from build123d import *

# Parameters (mm, degrees)
SKETCH1_W           = 18.495
SKETCH1_H           = 20.8
SKETCH1_W_2         = 10
SKETCH1_W_3         = 37.395
BOSS_EXTRUDE1_DEPTH = 10
SKETCH2_W           = 10
SKETCH2_H           = 20.8
BOSS_EXTRUDE2_DEPTH = 28.2
SKETCH6_W           = 106.79
SKETCH6_H           = 10
BOSS_EXTRUDE4_DEPTH = 10
SKETCH9_R           = 2.35
CUT_EXTRUDE1_DEPTH  = 10


with BuildPart() as part:
    # Sketch1 → Boss-Extrude1 (new body)
    with BuildSketch(Plane.XY):
        with Locations((-39.1475, 0)):
            Rectangle(SKETCH1_W, SKETCH1_H)
        with Locations((-53.395, 0)):
            Rectangle(SKETCH1_W_2, SKETCH1_H)
        with Locations((29.6975, 0)):
            Rectangle(SKETCH1_W_3, SKETCH1_H)
    extrude(amount=BOSS_EXTRUDE1_DEPTH)

    # Sketch2 → Boss-Extrude2 (add)
    with BuildSketch(Plane.XY.offset(10)):
        with Locations((43.395, 0)):
            Rectangle(SKETCH2_W, SKETCH2_H)
        with Locations((-53.395, 0)):
            Rectangle(SKETCH2_W, SKETCH2_H)
    extrude(amount=BOSS_EXTRUDE2_DEPTH)

    # Sketch6 → Boss-Extrude4 (add)
    with BuildSketch(Plane(origin=(0, 10.4, 0), x_dir=(1, 0, 0), z_dir=(0, 1, 0))):
        with Locations((-5, -5)):
            Rectangle(SKETCH6_W, SKETCH6_H)
    extrude(amount=BOSS_EXTRUDE4_DEPTH)

    # Sketch9 → Cut-Extrude1 (cut)
    with BuildSketch(Plane.XY.offset(10)):
        with Locations((14.89, -4.9)):
            Circle(SKETCH9_R)
        with Locations(Location((14.89, 4.9, 0), (0, 0, 180))):
            Circle(SKETCH9_R)
        with Locations(Location((-33.79, -4.9, 0), (0, 0, 180))):
            Circle(SKETCH9_R)
        with Locations((-33.79, 4.9)):
            Circle(SKETCH9_R)
    extrude(amount=-CUT_EXTRUDE1_DEPTH, mode=Mode.SUBTRACT)


solid = part.part
Verification items for the finished model (mm, model axes). A direction names the side the tool comes from. Coordinates: 2 decimals unless noted, no trailing zeros. Order: outer loops, then holes, each group sorted by start corner. A loop starts at its lowest first (then second) coordinate and runs counter-clockwise, first axis right, second up. Notation, with made-up numbers: M -25,82.25 L 4,82.25 A14 ccw 4,98.25 Z; hole C 36,1 d7. An arc over 180 degrees is marked long. One line per item, written item: value. Start each with the question number.
Item 1: Scan lines: probe 1 along Y at (x, z) = (14.89, 6.25); probe 2 along Y at (x, z) = (14, 2); probe 3 along X at (y, z) = (-4, 6) (3 decimals). Record each from-to range of solid material in increasing order.
Item 2: Gauge pin test, flat ends, axial feed: pin 1 (3 mm diameter, centred on x = 43.5, z = 23.5, fed in from +Y); pin 2 (8 mm diameter, centred on x = -24.5, z = 16.5, fed in from -Y); pin 3 (15.5 mm diameter, centred on x = -3.5, y = 11, fed in from +Z); pin 4 (8 mm diameter, centred on x = -3.5, z = 7.5, fed in from -Y). Record the tip position at first contact, or that the pin passes through.
Item 3: Sectioned sample at C-C (x = 16). Enter the section's corners in (y, z), then the cut area to 3 significant figures.
Item 4: Access from +Z, -Z, +X, -X, +Y, -Y to the whole of each face (thin tool, end or side, straight path). Record for faces 4 (the flat face through (-53, 10.4, 24)), 5 (the flat face through (11, 0, 5)), 6 (the flat face through (-48.395, 0, 24)), 7 (the cylindrical face through (-31.62, 4, 5.07)).
Item 5: Mould release check, pull along X, two halves, no side actions. Record for faces 1 (the flat face through (-10, 10.4, 5)), 2 (the flat face through (-58.395, 1, 19)), 3 (the flat face through (-51, -10.4, 15)): released by +X, released by -X, zero draft, split by the parting line, or undercut.
Item 6: Sectioned sample at D-D (y = -4.9). Enter the section's corners in (x, z) (3 decimals), then the cut area to 3 significant figures.
Item 7: Sectioned sample at B-B (z = 3). Enter the section's corners in (x, y) (3 decimals).
Item 8: Sectioned sample at A-A (y = 9). Enter the section's corners in (x, z) (3 decimals), then the cut area to 3 significant figures.
Conclusion:
1. probe 1: y = -10.4 to -7.25, -2.55 to 2.55, 7.25 to 20.4
1. probe 2: y = -10.4 to -7.07, -2.73 to 2.73, 7.07 to 20.4
1. probe 3: x = -58.395 to -35.961, -31.619 to -29.9, 11 to 12.719, 17.061 to 48.395
2. pin 1: stops at y = 10.4
2. pin 2: passes through
2. pin 3: stops at z = 10
2. pin 4: stops at y = 10.4
3. outline: M -10.4,0 L -6.97,0 L -6.97,10 L -10.4,10 Z; M -2.83,0 L 2.83,0 L 2.83,10 L -2.83,10 Z; M 6.97,0 L 20.4,0 L 20.4,10 L 6.97,10 Z
3. area: 225 mm^2
4. face 4: +Z, +X, -X, +Y
4. face 5: +Z, -Z, -Y
4. face 6: +Z, +Y, -Y
4. face 7: +Z, -Z
5. face 1: undercut
5. face 2: released by -X
5. face 3: zero draft
6. outline: M -58.395,0 L -36.14,0 L -36.14,10 L -48.395,10 L -48.395,38.2 L -58.395,38.2 Z; M -31.44,0 L -29.9,0 L -29.9,10 L -31.44,10 Z; M 11,0 L 12.54,0 L 12.54,10 L 11,10 Z; M 17.24,0 L 48.395,0 L 48.395,38.2 L 38.395,38.2 L 38.395,10 L 17.24,10 Z
6. area: 1,130 mm^2
7. outline: M -58.395,-10.4 L -29.9,-10.4 L -29.9,10.4 L 11,10.4 L 11,-10.4 L 48.395,-10.4 L 48.395,20.4 L -58.395,20.4 Z; hole C -33.79,-4.9 d4.7; hole C -33.79,4.9 d4.7; hole C 14.89,-4.9 d4.7; hole C 14.89,4.9 d4.7
8. outline: M -58.395,0 L -29.9,0 L -29.9,10 L -48.395,10 L -48.395,38.2 L -58.395,38.2 Z; M 11,0 L 48.395,0 L 48.395,38.2 L 38.395,38.2 L 38.395,10 L 11,10 Z
8. area: 1,220 mm^2
